Source: CAD feature listing. Evaluate the final solid. Frame: model axes, mm. A direction names the side the tool comes from. Round coordinates to 2 decimals unless told otherwise and drop trailing zeros. Loops run counter-clockwise (first coordinate to the right, second up) from the corner with the lowest first, then second, coordinate; pieces in that order, holes last. Notation, with made-up numbers: (-5, -31.5) -> (43, -31.5) arc R13 cw to (43, -10.5) -> close; hole circle Ø11 at (52, 76). An arc over 180 degrees is marked (long way). Return JSON: item names as keys, results as strings. Group by question number.
```python
from build123d import *

# Parameters (mm, degrees)
RESSALTO_EXTRUS_O2_DEPTH = 20
ESBO_O6_W                = 20
ESBO_O6_H                = 8
RESSALTO_EXTRUS_O3_DEPTH = 4
ESBO_O5_R                = 1.65
CORTE_EXTRUS_O2_DEPTH    = 27.773270252
FILETE1_R                = 1


with BuildPart() as part:
    # Esboço4 → Ressalto-extrusão2 (new body)
    with BuildSketch(Plane(origin=(0, 0, 0), x_dir=(0, 0, -1), z_dir=(1, 0, 0))):
        Polygon((0, 0), (15.92, 7.96), (15.92, 3.96), (8, 0), align=None)
    extrude(amount=RESSALTO_EXTRUS_O2_DEPTH)

    # Esboço6 → Ressalto-extrusão3 (add)
    with BuildSketch(Plane.XZ):
        with Locations((10, -4)):
            Rectangle(ESBO_O6_W, ESBO_O6_H)
    extrude(amount=-RESSALTO_EXTRUS_O3_DEPTH)

    # Esboço5 → Corte-extrusão2 (cut, through all)
    with BuildSketch(Plane.XZ):
        with Locations(Location((5, -4, 0), (0, 0, 270))):
            Circle(ESBO_O5_R)
        with Locations(Location((15, -4, 0), (0, 0, 270))):
            Circle(ESBO_O5_R)
    extrude(amount=-CORTE_EXTRUS_O2_DEPTH, mode=Mode.SUBTRACT)

    # Filete1
    filete1_edges = [part.edges().sort_by_distance(p)[0] for p in [
        (20, 5.98, -11.96),
        (0, 4, -4),
        (20, 4, -4),
        (20, 2, 0),
        (10, 4, 0),
        (0, 2, 0),
        (0, 5.98, -11.96),
        (0, 1.98, -11.96),
        (20, 1.98, -11.96),
    ]]
    fillet(filete1_edges, radius=FILETE1_R)


solid = part.part
```
(1) Cut plane A-A (x = 15). Return loops of the section in (y, z).
(2) Cut plane D-D (y = 1.75). Count the separate pieces of the cut face and the enclosed holes in it, and give its area (3 significant figures).
(3) Ray query, line 1 (X direction, y = 2.85, z = -4); line 2 (Y direction, x = 7.5, z = -1.5); line 3 (Z direction, x = 4.25, y = 1.75). Return the intervals inside material, ascending.
(4) Set-up query: faces 5 (the face through (0.285, 3.699, -4.567)), 6 (the face through (19.699, 3.715, -4.567)), 7 (the face through (10, 4, -4)), 8 (the face through (10, 1, 0)), 9 (the face through (0, 2, -7)). Return all of +Z, -Z, +X, -X, +Y, -Y with unobstructed straight access to the full face (end or side cutting, diameter ignored); none if empty.
(5) Cut plane C-C (x = 9). Return loops of the section in (y, z), and give its area (3 significant figures).
(6) Mould query, pull axis Z, two halves, no side actions, for faces 1 (the face through (0.285, 1.878, -11.084)), 2 (the face through (16.115, 1.972, -2.784)), 3 (the face through (3.4, 2, -3.6)), 4 (the face through (10, 0, -4)). Classes: released by +Z, released by -Z, zero draft, split by the parting line, or undercut.
(7) Cut plane B-B (z = -4). Return loops of the section in (x, y).
(8) Pin query (flat end, axial travel): pin 1 (1.5 mm diameter, centred on y = 6, z = -6, fed in from +X) (3 decimals); pin 2 (3 mm diameter, centred on x = 3.5, z = -13, fed in from -Y); pin 3 (2 mm diameter, centred on x = 10.5, z = -4.5, fed in from +Y); pin 4 (4.5 mm diameter, centred on x = 15, z = -4, fed in from -Y). Return the tip coordinate at first contact, or that it passes through.
Answers follow:
{
 "1": {"outline": "(0, -8) -> (3.96, -15.92) -> (7.96, -15.92) -> (4, -8) -> (4, -5.65) -> (0, -5.65) -> close; (0, -2.35) -> (4, -2.35) -> (4, -1) arc R1 ccw to (3, 0) -> (0, 0) -> close"},
 "2": {"separate pieces": "1", "enclosed holes": "2", "area": "212 mm^2"},
 "3": {"line 1": "0 to 3.35, 6.65 to 13.35, 16.65 to 20", "line 2": "0 to 4", "line 3": "-11.5 to -5.47, -2.53 to 0"},
 "4": {"face 5": "+Z, -X, +Y", "face 6": "+Z, +X, +Y", "face 7": "+Z, +X, -X, +Y", "face 8": "+Z, +X, -X, +Y, -Y", "face 9": "+Z, -Z, -X, +Y, -Y"},
 "5": {"outline": "(0, -8) -> (3.96, -15.92) -> (7.96, -15.92) -> (4, -8) -> (4, -1) arc R1 ccw to (3, 0) -> (0, 0) -> close", "area": "63.5 mm^2"},
 "6": {"face 1": "released by -Z", "face 2": "undercut", "face 3": "undercut", "face 4": "zero draft"},
 "7": {"outline": "(0, 0) -> (3.35, 0) -> (3.35, 4) -> (1, 4) arc R1 ccw to (0, 3) -> close; (6.65, 0) -> (13.35, 0) -> (13.35, 4) -> (6.65, 4) -> close; (16.65, 0) -> (20, 0) -> (20, 3) arc R1 ccw to (19, 4) -> (16.65, 4) -> close"},
 "8": {"pin 1": "through", "pin 2": "y = 1.75", "pin 3": "y = 4", "pin 4": "y = 0"}
}
